Geometry check sheet. Reference: drawing and pictorial views, mm from the part's lowest x, y, z. Round coordinates to 2 decimals unless told otherwise and drop trailing zeros. Loops run counter-clockwise (first coordinate to the right, second up) from the corner with the lowest first, then second, coordinate; pieces in that order, holes last. Notation, with made-up numbers: (66.5, 66) - (121.5, 66) arc R17 cw to (121.5, 76) - close; hole circle Ø4 at (-16.5, -35.75). An arc over 180 degrees is marked (long way). Put each result on its own line as item: value. Start each with the question number.
Item 1: Gauge pin test, flat end, axial feed: pin 1 Ø1.2 at (x, z) = (3.05, 3.05) entering from +Y. Record the tip position at first contact, or that the pin passes through.
Item 2: Section check C-C, the plane y = 0.7. Record the cut outline in (x, z).
Item 3: Material ranges on line 1 along X through (y, z) = (1.6, 3.05); line 2 along Z through (x, y) = (3.05, 0.5), recorded low to high.
Item 4: Draft check along X on the marked faces 1, 2 and 3. Enter one of: pulls with the +X half, pulls with the -X half, needs draft (parallel to the pull), parting line crosses it, or undercut.
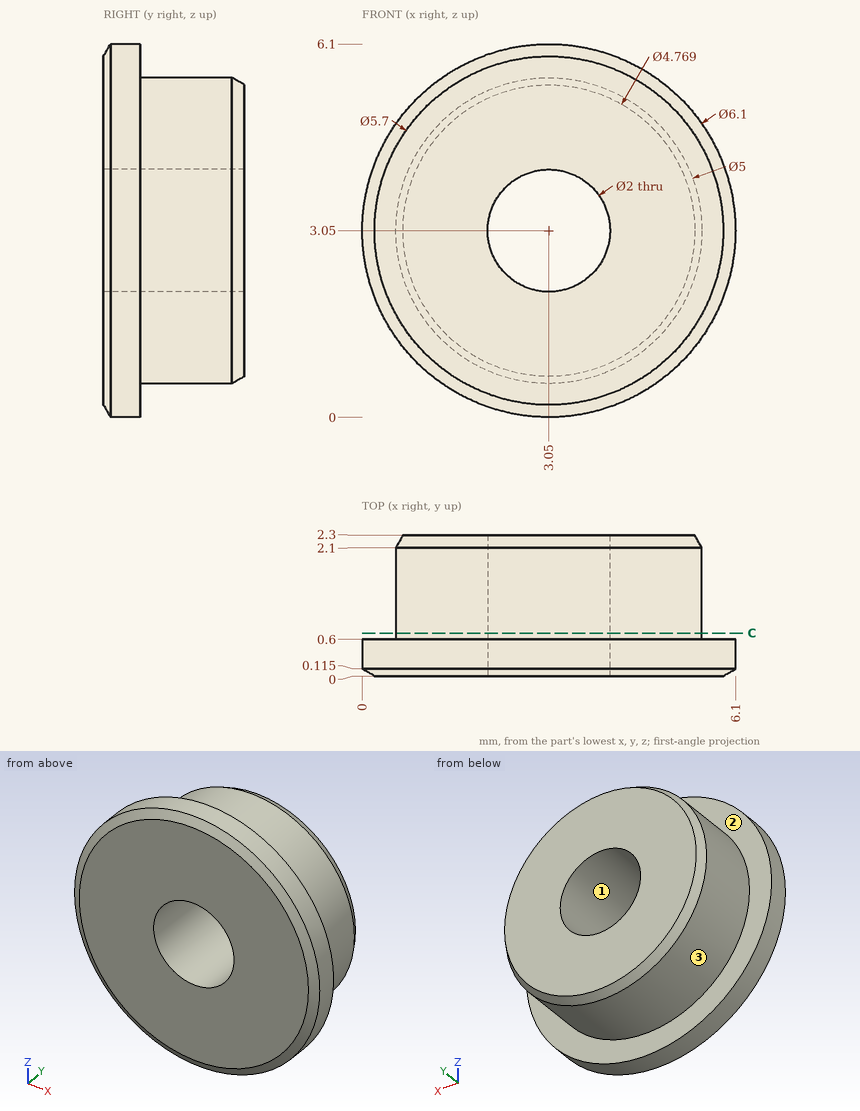
Check result:
1. pin 1: through
2. outline: circle Ø5 at (3.05, 3.05); hole circle Ø2 at (3.05, 3.05)
3. line 1: 0.55 to 2.05, 4.05 to 5.55
3. line 2: 0 to 2.05, 4.05 to 6.1
4. face 1: undercut
4. face 2: needs draft
4. face 3: parting line crosses it
